Build history of the part. All positions in model axes, mm. A direction names the side the tool comes from. Coordinates: 2 decimals unless noted, no trailing zeros. Write each loop counter-clockwise with the first axis right and the second up, starting at its lowest first coordinate (ties: lowest second). Pieces come first, ordered by that corner, then holes.
```python
from build123d import *


with BuildPart() as f2:
    # F2: sweep along a path in F1
    with BuildLine(Plane.XY) as f2_path:
        Line((-41.6680008888, 0), (-41.6680008888, 203.2))
        Line((-41.6680008888, 203.2), (-790.9680008888, 203.2))
        Line((-790.9680008888, 203.2), (-790.9680008888, -546.1))
        Line((-790.9680008888, -546.1), (-41.6680008888, -546.1))
        Line((-41.6680008888, -546.1), (-41.6680008888, -342.9))
    # F0 (on Front) → F2 (sweep)
    with BuildSketch(Plane.XZ):
        Polygon((0, 63.5), (-38.1, 63.5), (-38.1, 0), (-38.1, -63.5), (0, -63.5), (25.4, -38.1), (25.4, 0), (25.4, 38.1), align=None)
    sweep(path=f2_path.line, transition=Transition.RIGHT)


solid = f2.part
```
1. Mould opens along Y. For faces 1 (the face through (-6, 0, 1)), 2 (the face through (12.5, 137, -51)), 3 (the face through (-38.1, 105, 1)), 4 (the face through (-410.13, -600.29, -50.98)) say: +Y half, -Y half, draft (parallel to the pull), parting line (faces both ways), or undercut.
Computed values:
face 1: undercut
face 2: draft
face 3: undercut
face 4: -Y half
2. Probe line 1 along Y through (x, z) = (-221.5, 1); line 2 along X through (y, z) = (-360, 34); line 3 along X through (y, z) = (166.5, -51.5). List the from-to ranges inside material, lowest first.
Computed values:
line 1: y = -613.17 to -549.67, 206.77 to 270.27
line 2: x = -858.04 to -794.54, -38.1 to 25.4
line 3: x = -844.64 to -794.54, -38.1 to 12
3. Flat gauge pin, fed straight in: pin 1 (10 mm diameter, centred on y = -194.5, z = 20, fed in from +X). Where does the tip first touch, or does it go through?
Computed values:
pin 1: stops at x = -794.54
4. Saw through at A-A on y = 119.5. List the corners of the cut face in (x, z), plus the area to 3 significant figures.
Computed values:
outline: (-858.04, -38.1) - (-832.64, -63.5) - (-794.54, -63.5) - (-794.54, 63.5) - (-832.64, 63.5) - (-858.04, 38.1) - close; (-38.1, -63.5) - (0, -63.5) - (25.4, -38.1) - (25.4, 38.1) - (0, 63.5) - (-38.1, 63.5) - close
area: 14,800 mm2
5. Saw through at D-D on y = -135.5. List the corners of the cut face in (x, z), plus the area to 3 significant figures.
Computed values:
outline: (-858.04, -38.1) - (-832.64, -63.5) - (-794.54, -63.5) - (-794.54, 63.5) - (-832.64, 63.5) - (-858.04, 38.1) - close
area: 7,420 mm2
6. 3-axis set-ups, long thin cutter, end or side, ignore diameter. For faces 5 (the face through (-422, 206.768, 1)), 6 (the face through (-410, -613.168, -1)), 7 (the face through (-6, -342.9, 1)): which of +Z, -Z, +X, -X, +Y, -Y reach the whole face in a straight line?
Computed values:
face 5: +Z, -Z
face 6: +Z, -Z, +X, -X, -Y
face 7: +Z, -Z, +X
7. Saw through at C-C on z = -6. List the corners of the cut face in (x, y), plus the area to 3 significant figures.
Computed values:
outline: (-858.04, -613.17) - (25.4, -613.17) - (25.4, -342.9) - (-38.1, -342.9) - (-38.1, -549.67) - (-794.54, -549.67) - (-794.54, 206.77) - (-38.1, 206.77) - (-38.1, 0) - (25.4, 0) - (25.4, 270.27) - (-858.04, 270.27) - close
area: 186,000 mm2
8. Saw through at B-B on x = -679. List the corners of the cut face in (y, z).
Computed values:
outline: (-613.17, -38.1) - (-587.77, -63.5) - (-549.67, -63.5) - (-549.67, 63.5) - (-587.77, 63.5) - (-613.17, 38.1) - close; (206.77, -63.5) - (244.87, -63.5) - (270.27, -38.1) - (270.27, 38.1) - (244.87, 63.5) - (206.77, 63.5) - close
